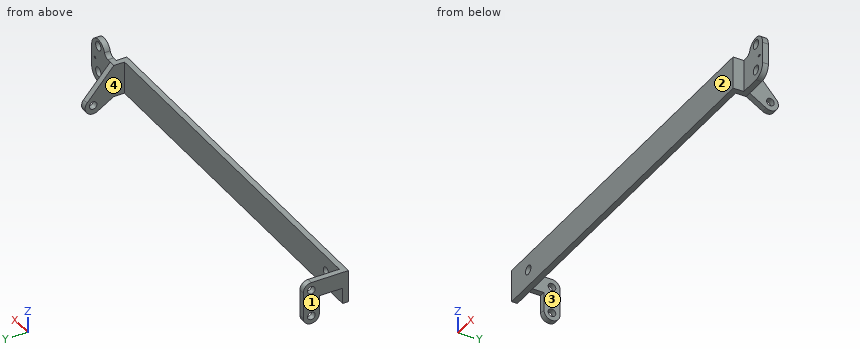
```python
from build123d import *

# Parameters (mm, degrees)
EXTRUDE_THIN1_DEPTH = 85
BOSS_EXTRUDE1_DEPTH = 15
BOSS_EXTRUDE2_DEPTH = 16
FILLET1_R           = 21
BOSS_EXTRUDE3_DEPTH = 15
FILLET2_R           = 16
SKETCH6_R           = 12
CUT_EXTRUDE2_DEPTH  = 1094.547438386
FILLET3_R           = 30
SKETCH7_R           = 12
CUT_EXTRUDE3_DEPTH  = 1096.823890961
SKETCH9_R           = 10
CUT_EXTRUDE4_DEPTH  = 1098.335409071
CUT_EXTRUDE5_DEPTH  = 1094.547438386


with BuildPart() as part:
    # Sketch1 → Extrude-Thin1 (new body)
    with BuildSketch(Plane.XY):
        Polygon((0, 0), (1000, 0), (1000, 28), (1085, 28), (1085, 43), (985, 43), (985, 15), (0, 15), align=None)
    extrude(amount=-EXTRUDE_THIN1_DEPTH)

    # Sketch2 → Boss-Extrude1 (add)
    with BuildSketch(Plane.ZY):
        Polygon((0, 15), (0, 118), (-112, 118), (-112, 76), (-43, 76), (-43, 15), align=None)
    extrude(amount=-BOSS_EXTRUDE1_DEPTH)

    # Sketch3 → Boss-Extrude2 (add)
    with BuildSketch(Plane.ZY.offset(-985)):
        with BuildLine():
            Line((0, 43), (-79.111854281, 112.751806515))
            ThreePointArc((-79.111854281, 112.751806515), (-106.449245092, 113.128168106), (-110.990788091, 86.168031394))
            Line((-110.990788091, 86.168031394), (-85, 43))
            Line((-85, 43), (0, 43))
        make_face()
    extrude(amount=-BOSS_EXTRUDE2_DEPTH)

    # Fillet1
    fillet1_edges = [part.edges().sort_by_distance(p)[0] for p in [
        (7.5, 76, -112),
        (7.5, 118, -112),
        (7.5, 118, 0),
    ]]
    fillet(fillet1_edges, radius=FILLET1_R - 0.0001)  # a hair under: the kernel refuses the full size

    # Sketch5 → Boss-Extrude3 (add)
    with BuildSketch(Plane(origin=(0, 43, 0), x_dir=(1, 0, 0), z_dir=(0, 1, 0))):
        with BuildLine():
            Line((1025, 0), (1085, 0))
            ThreePointArc((1085, 0), (1055, -30), (1025, 0))
        make_face()
    extrude(amount=-BOSS_EXTRUDE3_DEPTH)

    # Fillet2
    fillet2_edges = [part.edges().sort_by_distance(p)[0] for p in [
        (1025, 35.5, 0),
    ]]
    fillet(fillet2_edges, radius=FILLET2_R)

    # Sketch6 → Cut-Extrude2 (cut, through all)
    with BuildSketch(Plane(origin=(0, 43, 0), x_dir=(1, 0, 0), z_dir=(0, 1, 0))):
        with Locations(Location((1055, -12, 0), (0, 0, 270))):
            Circle(SKETCH6_R)
        with Locations(Location((1055, 58, 0), (0, 0, 270))):
            Circle(SKETCH6_R)
    extrude(amount=-CUT_EXTRUDE2_DEPTH, mode=Mode.SUBTRACT)

    # Fillet3
    fillet3_edges = [part.edges().sort_by_distance(p)[0] for p in [
        (1085, 35.5, -85),
    ]]
    fillet(fillet3_edges, radius=FILLET3_R)

    # Sketch7 → Cut-Extrude3 (cut, through all)
    with BuildSketch(Plane(origin=(0, 15, 0), x_dir=(1, 0, 0), z_dir=(0, 1, 0))):
        with Locations(Location((75, 42, 0), (0, 0, 270))):
            Circle(SKETCH7_R)
    extrude(amount=-CUT_EXTRUDE3_DEPTH, mode=Mode.SUBTRACT)

    # Sketch9 → Cut-Extrude4 (cut, through all)
    with BuildSketch(Plane.ZY):
        with Locations((-91, 97)):
            Circle(SKETCH9_R)
        with Locations((-21, 97)):
            Circle(SKETCH9_R)
    extrude(amount=-CUT_EXTRUDE4_DEPTH, mode=Mode.SUBTRACT)

    # Sketch10 → Cut-Extrude5 (cut, through all)
    with BuildSketch(Plane(origin=(0, 43, 0), x_dir=(1, 0, 0), z_dir=(0, 1, 0))):
        with BuildLine():
            Line((1067.041960108, 28), (1072.958039892, 28))
            ThreePointArc((1072.958039892, 28), (1070, 30.5), (1067.041960108, 28))
        make_face()
        with BuildLine():
            ThreePointArc((1067.041960108, 27), (1070, 24.5), (1072.958039892, 27))
            Line((1072.958039892, 27), (1067.041960108, 27))
        make_face()
        with BuildLine():
            Line((1075, 27), (1075, 28))
            Line((1075, 28), (1072.958039892, 28))
            ThreePointArc((1072.958039892, 28), (1072.989491568, 27.750878781), (1073, 27.5))
            ThreePointArc((1073, 27.5), (1072.989491568, 27.249121219), (1072.958039892, 27))
            Line((1072.958039892, 27), (1075, 27))
        make_face()
        with BuildLine():
            ThreePointArc((1067.041960108, 27), (1067, 27.5), (1067.041960108, 28))
            Line((1067.041960108, 28), (1065, 28))
            Line((1065, 28), (1065, 27))
            Line((1065, 27), (1067.041960108, 27))
        make_face()
        with BuildLine():
            ThreePointArc((1073, 27.5), (1072.989491568, 27.750878781), (1072.958039892, 28))
            Line((1072.958039892, 28), (1067.041960108, 28))
            ThreePointArc((1067.041960108, 28), (1067, 27.5), (1067.041960108, 27))
            Line((1067.041960108, 27), (1072.958039892, 27))
            ThreePointArc((1072.958039892, 27), (1072.989491568, 27.249121219), (1073, 27.5))
        make_face()
    extrude(amount=-CUT_EXTRUDE5_DEPTH, mode=Mode.SUBTRACT)


solid = part.part
```
Design review of the part built by this model. Coordinates are the model's own, in mm. Face numbers are marked on the shaded views. Coordinates: 2 decimals unless noted, no trailing zeros. Order: outer loops, then holes, each group sorted by start corner. A loop starts at its lowest first (then second) coordinate and runs counter-clockwise, first axis right, second up. Notation, with made-up numbers: M 49.5,68.25 L 92.5,68.25 A24 cw 92.5,102.25 Z; hole C 75.5,26 d1. An arc over 180 degrees is marked long. Answer as a JSON object with one key per item and string values. Group by question number.
1) Add section C-C, the plane x = 509. Write out the cut boundary in (y, z).
2) Mouldability with a two-part tool opening along X and no side actions: class the marked faces 1, 2, 3 and 4 as pulls with the +X half, pulls with the -X half, needs draft (parallel to the pull), parting line crosses it, or undercut.
3) Add section A-A, the plane x = 75. Write out the cut boundary in (y, z).
4) For pin 1 (1 mm diameter, centred on x = 1065.5, y = 34, fed in from +Z); pin 2 (21.5 mm diameter, centred on x = 515.5, y = 20.5, fed in from -Z); pin 3 (5 mm diameter, centred on y = 71.5, z = -41.5, fed in from +X), all flat-tipped, find the tip position at first contact; note any pin that passes through.
5) Wall thickness on L1, parallel to Z at x = 1055, y = 35; L2, parallel to X at y = 33, z = -7.5; L3, parallel to X at y = 44.5, z = -16.5: over which ranges is each line inside the solid? List them lowest first.
6) Add section B-B, the plane y = 64.5. Write out the cut boundary in (x, z).
Computed values:
{
 "1": {"outline": "M 0,-85 L 15,-85 L 15,0 L 0,0 Z"},
 "2": {"face 1": "pulls with the -X half", "face 2": "needs draft", "face 3": "undercut", "face 4": "undercut"},
 "3": {"outline": "M 0,-85 L 15,-85 L 15,-54 L 0,-54 Z; M 0,-30 L 15,-30 L 15,0 L 0,0 Z"},
 "4": {"pin 1": "stops at z = 28.28", "pin 2": "stops at z = -85", "pin 3": "stops at x = 1001"},
 "5": {"L1": "z = -85 to -70, -46 to 0, 24 to 30", "L2": "x = 0 to 15, 985 to 1085", "L3": "x = 0 to 15, 985 to 1001"},
 "6": {"outline": "M 0,-43 L 15,-43 L 15,0 L 0,0 Z; M 985,-97.94 L 1001,-97.94 L 1001,-24.39 L 985,-24.39 Z"}
}
